The listing builds one solid part. Answer for the finished solid, in the listing's coordinates (mm). A direction names the side the tool comes from. Coordinates: 2 decimals unless noted, no trailing zeros. Loops run counter-clockwise (first coordinate to the right, second up) from the corner with the lowest first, then second, coordinate; pieces in that order, holes last. Notation, with made-up numbers: M -4,50 L 15,50 A11 cw 15,70 Z; hole C 24,5.5 d11. An arc over 180 degrees is marked long. Return JSON: item names as keys, results as strings. Group by question number.
1. Section B-B (z = -13) is taken. Write down the section's boundary in (x, y), then the cut area to 3 significant figures.
2. Section D-D (y = 3.5) is taken. Write down the section's boundary in (x, z), then the cut area to 3 significant figures.
3. Which of the six approach directions +Z, -Z, +X, -X, +Y, -Y give full straight-line access (tool end or side, diameter ignored) to faces 1 (the face through (-40, 11, -38.1)), 2 (the face through (-31.67, 24.76, -19.59))?
4. Section A-A (y = 18.25) is taken. Write down the section's boundary in (x, z).
5. Given P1, Ø8, axis at x = -56.5, z = -33.5, coming from the -Y side; P2, Ø10.5, axis at x = -41.5, z = -24, coming from the -Y side; P3, Ø1.4, axis at x = -1, y = 8.5, coming from the -Z side; P4, Ø1.4, axis at x = -1, z = -20, coming from the -Y side, each flat-ended and moving along its own axis, determine where each tip first touches the part or whether it passes through.
6. The mould has two halves that part along Z. Classify faces 3 (the face through (-38.854, 24.636, -0.724)), 4 (the face through (-0.724, 24.636, -19.925)), 5 (the face through (-1.27, 14, -19)), 6 (the face through (-77.47, 11, -19)): pulls with the +Z half, pulls with the -Z half, needs draft (parallel to the pull), parting line crosses it, or undercut.
7. Straight lines are drawn through the part: L1, parallel to Z at x = -53.5, y = 12.5; L2, parallel to X at y = 9.5, z = -29; L3, parallel to X at y = 6, z = -21.5. For each, find the intervals that lie inside material, in ascending order. Write a range as from..to.
8. Section C-C (x = -53.5) is taken. Write down the section's boundary in (y, z), then the cut area to 3 significant figures.
```python
from build123d import *

# Parameters (mm, degrees)
SKETCH1_W           = 78.74
SKETCH1_H           = 39.37
BOSS_EXTRUDE1_DEPTH = 25.4
FILLET1_R           = 2.54
SHELL1_T            = -1.27
SKETCH2_R           = 8.5979
CUT_EXTRUDE1_DEPTH  = 92.281111956
SKETCH3_W           = 15.875
SKETCH3_H           = 8.89
CUT_EXTRUDE2_DEPTH  = 1.27


with BuildPart() as part:
    # Sketch1 → Boss-Extrude1 (new body)
    with BuildSketch(Plane(origin=(0, 0, 0), x_dir=(1, 0, 0), z_dir=(0, 1, 0))):
        with Locations((-39.37, 19.685)):
            Rectangle(SKETCH1_W, SKETCH1_H)
    extrude(amount=BOSS_EXTRUDE1_DEPTH)

    # Fillet1
    fillet1_edges = [part.edges().sort_by_distance(p)[0] for p in [
        (-78.74, 25.4, -19.685),
        (-39.37, 25.4, 0),
        (0, 25.4, -19.685),
        (-39.37, 25.4, -39.37),
        (0, 12.7, 0),
        (-78.74, 12.7, 0),
        (-78.74, 12.7, -39.37),
        (0, 12.7, -39.37),
    ]]
    fillet(fillet1_edges, radius=FILLET1_R)

    # Shell1
    shell1_openings = [part.faces().sort_by_distance(p)[0] for p in [
        (-39.37, 0, -19.685),
    ]]
    offset(amount=SHELL1_T, openings=shell1_openings, kind=Kind.INTERSECTION)

    # Sketch2 → Cut-Extrude1 (cut, through all)
    with BuildSketch(Plane.XZ.offset(-24.13)):
        with Locations(Location((-52.2986, -26.416, 0), (0, 0, 270))):
            Circle(SKETCH2_R)
        with Locations(Location((-26.4414, -26.416, 0), (0, 0, 270))):
            Circle(SKETCH2_R)
    extrude(amount=-CUT_EXTRUDE1_DEPTH, mode=Mode.SUBTRACT)

    # Sketch3 → Cut-Extrude2 (cut)
    with BuildSketch(Plane(origin=(0, 0, 0), x_dir=(0, 0, -1), z_dir=(1, 0, 0))):
        with Locations((19.685, 6.985)):
            Rectangle(SKETCH3_W, SKETCH3_H)
    extrude(amount=-CUT_EXTRUDE2_DEPTH, mode=Mode.SUBTRACT)


solid = part.part
```
Worked out:
{
 "1": {"outline": "M -78.74,0 L -77.47,0 L -77.47,22.86 A1.27 cw -76.2,24.13 L -2.54,24.13 A1.27 cw -1.27,22.86 L -1.27,11.43 L 0,11.43 L 0,22.86 A2.54 ccw -2.54,25.4 L -76.2,25.4 A2.54 ccw -78.74,22.86 Z; M -1.27,0 L 0,0 L 0,2.54 L -1.27,2.54 Z", "area": "148 mm^2"},
 "2": {"outline": "M -78.74,-36.83 A2.54 ccw -76.2,-39.37 L -2.54,-39.37 A2.54 ccw 0,-36.83 L 0,-27.62 L -1.27,-27.62 L -1.27,-36.83 A1.27 cw -2.54,-38.1 L -76.2,-38.1 A1.27 cw -77.47,-36.83 L -77.47,-2.54 A1.27 cw -76.2,-1.27 L -2.54,-1.27 A1.27 cw -1.27,-2.54 L -1.27,-11.75 L 0,-11.75 L 0,-2.54 A2.54 ccw -2.54,0 L -76.2,0 A2.54 ccw -78.74,-2.54 Z", "area": "269 mm^2"},
 "3": {"face 1": "-Y", "face 2": "+Y, -Y"},
 "4": {"outline": "M -78.74,-36.83 A2.54 ccw -76.2,-39.37 L -2.54,-39.37 A2.54 ccw 0,-36.83 L 0,-2.54 A2.54 ccw -2.54,0 L -76.2,0 A2.54 ccw -78.74,-2.54 Z; hole M -77.47,-36.83 A1.27 ccw -76.2,-38.1 L -2.54,-38.1 A1.27 ccw -1.27,-36.83 L -1.27,-2.54 A1.27 ccw -2.54,-1.27 L -76.2,-1.27 A1.27 ccw -77.47,-2.54 Z"},
 "5": {"P1": "y = 23.94", "P2": "y = 24.13", "P3": "z = -39.23", "P4": "y = 0"},
 "6": {"face 3": "pulls with the +Z half", "face 4": "needs draft", "face 5": "undercut", "face 6": "undercut"},
 "7": {"L1": "-39.37..-38.1, -1.27..0", "L2": "-78.74..-77.47, -1.27..0", "L3": "-78.74..-77.47"},
 "8": {"outline": "M 0,-39.37 L 22.86,-39.37 A2.54 ccw 25.4,-36.83 L 25.4,-34.93 L 24.13,-34.93 L 24.13,-36.83 A1.27 cw 22.86,-38.1 L 0,-38.1 Z; M 0,-1.27 L 22.86,-1.27 A1.27 cw 24.13,-2.54 L 24.13,-17.9 L 25.4,-17.9 L 25.4,-2.54 A2.54 ccw 22.86,0 L 0,0 Z", "area": "87.6 mm^2"}
}
